Here's how the part is built. I have some questions about the finished solid (model axes, mm). A direction names the side the tool comes from. Round coordinates to 2 decimals unless told otherwise and drop trailing zeros. Write each loop counter-clockwise with the first axis right and the second up, starting at its lowest first coordinate (ties: lowest second). Pieces come first, ordered by that corner, then holes. Notation, with made-up numbers: (34, 67.5) - (63, 67.5) arc R31 cw to (63, 97.5) - close; hole circle Ø10 at (-25.75, 76.25). An arc over 180 degrees is marked (long way). One line per question, with ' | ' between items. Start each with the question number.
(1) For faces 3 (the flat face through (0, 25, 0.5)), 4 (the cylindrical face through (-2.38, 40.74, -1.27)), 5 (the flat face through (7, 35, -2.5)), 6 (the flat face through (5, -1, -2)), which set-ups out of +Z, -Z, +X, -X, +Y, -Y let a thin tool reach every point of the face, with its end or its side?
(2) Imagine slicing it at B-B (y = -26.6). Write out the boundary of the cut face in (x, z).
(3) Imagine slicing it at C-C (y = 16). Write out the boundary of the cut face in (x, z), plus the area to 3 significant figures.
(4) Imagine slicing it at D-D (x = -2). Write out the boundary of the cut face in (y, z), plus the area to 3 significant figures.
(5) Imagine slicing it at A-A (z = 4.25). Write out the boundary of the cut face in (x, y).
(6) Will these pins go through, and if not, where does the flat tip stop? pin 1 (4.5 mm diameter, centred on x = -8, y = -26.6, fed in from -Z); pin 2 (0.6 mm diameter, centred on x = 3.5, z = 0.5, fed in from +Y); pin 3 (2.5 mm diameter, centred on x = 5.66, y = 35.66, fed in from -Z); pin 4 (2.5 mm diameter, centred on x = -5.66, y = 35.66, fed in from +Z).
(7) If I drill on L1, parallel to Y at x = 0, z = 0.3; L2, parallel to Y at x = -0.75, z = -0.5; L3, parallel to Y at x = -1.5, z = 2, over which ranges is the centre line in solid material (lowest first)?
(8) Thinking about a two-plate mould opening in Y: for faces 1 (the flat face through (-0.2, -28.3, 5)), 2 (the cylindrical face through (-0.1, 18.5, -1.5)), which applies, pulls with the +Y half, pulls with the -Y half, needs draft (parallel to the pull), parting line crosses it, or undercut?
from build123d import *
from build123d.topology import SkipClean

# Parameters (mm, degrees)
BOSS_EXTRUDE1_DEPTH           = 3
BOSS_EXTRUDE2_START           = -0.5
SKETCH1_3_R                   = 11
BOSS_EXTRUDE2_DEPTH           = 0.5
SKETCH2_R                     = 4.1
SKETCH2_R_2                   = 1.1
CUT_EXTRUDE1_DEPTH            = 3.5
SKETCH2_3_R                   = 2
CUT_EXTRUDE2_DEPTH            = 0.5
CIRPATTERN2_COUNT             = 4
SKETCH1_6_W                   = 11
SKETCH1_6_H                   = 6
BOSS_EXTRUDE3_DEPTH           = 5
SKETCH4_R                     = 1.35
CUT_EXTRUDE4_DEPTH            = 8
LPATTERN2_COUNT               = 2
LPATTERN2_PITCH               = 8
LPATTERN2_COL_COUNT           = 2
LPATTERN2_COL_PITCH           = 8
BODY_MOVE_COPY1_START         = -3
BODY_MOVE_COPY1_OUTLINE_R     = 2
BODY_MOVE_COPY1_OUTLINE_R_2   = 4.1
BODY_MOVE_COPY1_DEPTH         = 3
BODY_MOVE_COPY1_START_2       = 3
BODY_MOVE_COPY1_2_OUTLINE_W   = 22
BODY_MOVE_COPY1_2_OUTLINE_H   = 6
BODY_MOVE_COPY1_2_OUTLINE_R   = 1.35
BODY_MOVE_COPY1_2_DEPTH       = 2
BODY_MOVE_COPY1_START_3       = -2.5
BODY_MOVE_COPY1_3_OUTLINE_R   = 2
BODY_MOVE_COPY1_3_OUTLINE_R_2 = 1.1
BODY_MOVE_COPY1_3_DEPTH       = 2
BODY_MOVE_COPY1_START_4       = 0.5
BODY_MOVE_COPY1_4_OUTLINE_R   = 1.1
BODY_MOVE_COPY1_4_OUTLINE_R_2 = 4.1
BODY_MOVE_COPY1_4_DEPTH       = 2.5
BODY_MOVE_COPY1_5_DEPTH       = 0.5
BODY_MOVE_COPY1_START_5       = -5
BODY_MOVE_COPY1_6_OUTLINE_W   = 22
BODY_MOVE_COPY1_6_OUTLINE_H   = 6
BODY_MOVE_COPY1_6_OUTLINE_R   = 1.35
BODY_MOVE_COPY1_6_DEPTH       = 2


# Read off the part's stored shape, not the designer's step: Body-Move/Copy1
with BuildPart() as part:
    # Sketch1 → Boss-Extrude1 (new body)
    with BuildSketch(Plane.XY):
        with BuildLine():
            Line((-11, 30), (-11, -30))
            Line((-11, -30), (11, -30))
            Line((11, -30), (11, 30))
            ThreePointArc((11, 30), (0, 41), (-11, 30))
        make_face()
        with BuildLine():
            Line((5, -23), (-5, -23))
            Line((-5, -23), (-5, 19.643842411))
            ThreePointArc((-5, 19.643842411), (0, 18.5), (5, 19.643842411))
            Line((5, 19.643842411), (5, -23))
        make_face(mode=Mode.SUBTRACT)
    extrude(amount=BOSS_EXTRUDE1_DEPTH)

    # Sketch1<3> → Boss-Extrude2 (add)
    with BuildSketch(Plane.XY.offset(BOSS_EXTRUDE2_START)):
        with Locations((0, 30)):
            Circle(SKETCH1_3_R)
    extrude(amount=BOSS_EXTRUDE2_DEPTH)

    # Sketch2 → Cut-Extrude1 (cut)
    with BuildSketch(Plane.XY.offset(3)):
        with Locations((0, 30)):
            Circle(SKETCH2_R)
        with Locations((5.656854249, 35.656854249)):
            Circle(SKETCH2_R_2)
    cut_extrude1 = extrude(amount=-CUT_EXTRUDE1_DEPTH, mode=Mode.SUBTRACT)

    # Sketch2<3> → Cut-Extrude2 (cut)
    with BuildSketch(Plane.XY.offset(3)):
        with Locations((5.656854249, 35.656854249)):
            Circle(SKETCH2_3_R)
    cut_extrude2 = extrude(amount=-CUT_EXTRUDE2_DEPTH, mode=Mode.SUBTRACT)

    # CirPattern2: Cut-Extrude1, Cut-Extrude2 ×4 about axis
    cirpattern2_axis = Axis((0, 30, 0), (0, 0, 1))
    add([cut_extrude1.rotate(cirpattern2_axis, i * 360 / CIRPATTERN2_COUNT) for i in range(1, CIRPATTERN2_COUNT)], mode=Mode.SUBTRACT)
    add([cut_extrude2.rotate(cirpattern2_axis, i * 360 / CIRPATTERN2_COUNT) for i in range(1, CIRPATTERN2_COUNT)], mode=Mode.SUBTRACT)

    # Sketch1<6> → Boss-Extrude3 (add)
    with BuildSketch(Plane.XY):
        with Locations((-5.5, -27)):
            Rectangle(SKETCH1_6_W, SKETCH1_6_H)
        with Locations((5.5, -27)):
            Rectangle(SKETCH1_6_W, SKETCH1_6_H)
    extrude(amount=-BOSS_EXTRUDE3_DEPTH)

    # Sketch4 → Cut-Extrude4 (cut)
    with BuildSketch(Plane.XY.offset(3)):
        with Locations((0, -26.6)):
            Circle(SKETCH4_R)
    cut_extrude4 = extrude(amount=-CUT_EXTRUDE4_DEPTH, mode=Mode.SUBTRACT)

    # LPattern2: Cut-Extrude4 ×2
    with Locations(*[(i * LPATTERN2_PITCH, 0, 0) for i in range(1, LPATTERN2_COUNT)]):
        add(cut_extrude4, mode=Mode.SUBTRACT)

    # LPattern2 col: Cut-Extrude4 ×2
    with Locations(*[(-i * LPATTERN2_COL_PITCH, 0, 0) for i in range(1, LPATTERN2_COL_COUNT)]):
        add(cut_extrude4, mode=Mode.SUBTRACT)

    # Body-Move/Copy1 outline → Body-Move/Copy1 (add)
    with BuildSketch(Plane.XY.offset(BODY_MOVE_COPY1_START)):
        with BuildLine():
            Line((-11, -24), (11, -24))
            Line((11, -24), (11, 30))
            ThreePointArc((11, 30), (0, 41), (-11, 30))
            Line((-11, 30), (-11, -24))
        make_face()
        with BuildLine():
            Line((5, 19.643842411), (5, -23))
            Line((5, -23), (-5, -23))
            Line((-5, -23), (-5, 19.643842411))
            ThreePointArc((-5, 19.643842411), (0, 18.5), (5, 19.643842411))
        make_face(mode=Mode.SUBTRACT)
        with Locations((5.656854249, 35.656854249)):
            Circle(BODY_MOVE_COPY1_OUTLINE_R, mode=Mode.SUBTRACT)
        with Locations((-5.656854249, 24.343145751)):
            Circle(BODY_MOVE_COPY1_OUTLINE_R, mode=Mode.SUBTRACT)
        with Locations((-5.656854249, 35.656854249)):
            Circle(BODY_MOVE_COPY1_OUTLINE_R, mode=Mode.SUBTRACT)
        with Locations((0, 30)):
            Circle(BODY_MOVE_COPY1_OUTLINE_R_2, mode=Mode.SUBTRACT)
        with Locations((5.656854249, 24.343145751)):
            Circle(BODY_MOVE_COPY1_OUTLINE_R, mode=Mode.SUBTRACT)
    extrude(amount=BODY_MOVE_COPY1_DEPTH)

    # Body-Move_Copy1 2 outline → Body-Move_Copy1 2 (add)
    with BuildSketch(Plane.XY.offset(BODY_MOVE_COPY1_START_2)):
        with Locations((0, -27)):
            Rectangle(BODY_MOVE_COPY1_2_OUTLINE_W, BODY_MOVE_COPY1_2_OUTLINE_H)
        with Locations((-8, -26.6)):
            Circle(BODY_MOVE_COPY1_2_OUTLINE_R, mode=Mode.SUBTRACT)
        with Locations((0, -26.6)):
            Circle(BODY_MOVE_COPY1_2_OUTLINE_R, mode=Mode.SUBTRACT)
        with Locations((8, -26.6)):
            Circle(BODY_MOVE_COPY1_2_OUTLINE_R, mode=Mode.SUBTRACT)
    extrude(amount=BODY_MOVE_COPY1_2_DEPTH)

    # Body-Move_Copy1 3 outline → Body-Move_Copy1 3 (add)
    # profile 1 of 4: a face of its own
    with BuildSketch(Plane.XY.offset(BODY_MOVE_COPY1_START_3)):
        with Locations((5.656854249, 35.656854249)):
            Circle(BODY_MOVE_COPY1_3_OUTLINE_R)
        with Locations((5.656854249, 35.656854249)):
            Circle(BODY_MOVE_COPY1_3_OUTLINE_R_2, mode=Mode.SUBTRACT)
    # profile 2 of 4: a face of its own
    with BuildSketch(Plane.XY.offset(BODY_MOVE_COPY1_START_3)):
        with Locations((5.656854249, 24.343145751)):
            Circle(BODY_MOVE_COPY1_3_OUTLINE_R)
        with Locations((5.656854249, 24.343145751)):
            Circle(BODY_MOVE_COPY1_3_OUTLINE_R_2, mode=Mode.SUBTRACT)
    # profile 3 of 4: a face of its own
    with BuildSketch(Plane.XY.offset(BODY_MOVE_COPY1_START_3)):
        with Locations((-5.656854249, 35.656854249)):
            Circle(BODY_MOVE_COPY1_3_OUTLINE_R)
        with Locations((-5.656854249, 35.656854249)):
            Circle(BODY_MOVE_COPY1_3_OUTLINE_R_2, mode=Mode.SUBTRACT)
    # profile 4 of 4: a face of its own
    with BuildSketch(Plane.XY.offset(BODY_MOVE_COPY1_START_3)):
        with Locations((-5.656854249, 24.343145751)):
            Circle(BODY_MOVE_COPY1_3_OUTLINE_R)
        with Locations((-5.656854249, 24.343145751)):
            Circle(BODY_MOVE_COPY1_3_OUTLINE_R_2, mode=Mode.SUBTRACT)
    extrude(amount=BODY_MOVE_COPY1_3_DEPTH)

    # Body-Move_Copy1 4 outline → Body-Move_Copy1 4 (cut)
    with BuildSketch(Plane.XY.offset(BODY_MOVE_COPY1_START_4)):
        with BuildLine():
            ThreePointArc((11, 30), (0, 41), (-11, 30))
            Line((-11, 30), (-11, -24))
            Line((-11, -24), (11, -24))
            Line((11, -24), (11, 30))
        make_face()
        with Locations((5.656854249, 35.656854249)):
            Circle(BODY_MOVE_COPY1_4_OUTLINE_R, mode=Mode.SUBTRACT)
        with Locations((0, 30)):
            Circle(BODY_MOVE_COPY1_4_OUTLINE_R_2, mode=Mode.SUBTRACT)
        with BuildLine():
            Line((5, -23), (-5, -23))
            Line((-5, -23), (-5, 19.643842411))
            ThreePointArc((-5, 19.643842411), (0, 18.5), (5, 19.643842411))
            Line((5, 19.643842411), (5, -23))
        make_face(mode=Mode.SUBTRACT)
        with Locations((-5.656854249, 24.343145751)):
            Circle(BODY_MOVE_COPY1_4_OUTLINE_R, mode=Mode.SUBTRACT)
        with Locations((-5.656854249, 35.656854249)):
            Circle(BODY_MOVE_COPY1_4_OUTLINE_R, mode=Mode.SUBTRACT)
        with Locations((5.656854249, 24.343145751)):
            Circle(BODY_MOVE_COPY1_4_OUTLINE_R, mode=Mode.SUBTRACT)
    extrude(amount=BODY_MOVE_COPY1_4_DEPTH, mode=Mode.SUBTRACT)

    # Body-Move_Copy1 5 outline → Body-Move_Copy1 5 (cut)
    with SkipClean():  # the faces are left unmerged after this step: merging them gives an invalid solid
        with BuildSketch(Plane.XY):
            with BuildLine():
                Line((-11, -24), (11, -24))
                Line((11, -24), (11, 30))
                ThreePointArc((11, 30), (0, 19), (-11, 30))
                Line((-11, 30), (-11, -24))
            make_face()
            with BuildLine():
                Line((5, 19.643842411), (5, -23))
                Line((5, -23), (-5, -23))
                Line((-5, -23), (-5, 19.643842411))
                ThreePointArc((-5, 19.643842411), (0, 18.5), (5, 19.643842411))
            make_face(mode=Mode.SUBTRACT)
        extrude(amount=BODY_MOVE_COPY1_5_DEPTH, mode=Mode.SUBTRACT)
    add(part.part.scale(1), mode=Mode.REPLACE)  # the faces are merged on a copy

    # Body-Move_Copy1 6 outline → Body-Move_Copy1 6 (cut)
    with BuildSketch(Plane.XY.offset(BODY_MOVE_COPY1_START_5)):
        with Locations((0, -27)):
            Rectangle(BODY_MOVE_COPY1_6_OUTLINE_W, BODY_MOVE_COPY1_6_OUTLINE_H)
        with Locations((-8, -26.6)):
            Circle(BODY_MOVE_COPY1_6_OUTLINE_R, mode=Mode.SUBTRACT)
        with Locations((0, -26.6)):
            Circle(BODY_MOVE_COPY1_6_OUTLINE_R, mode=Mode.SUBTRACT)
        with Locations((8, -26.6)):
            Circle(BODY_MOVE_COPY1_6_OUTLINE_R, mode=Mode.SUBTRACT)
    extrude(amount=BODY_MOVE_COPY1_6_DEPTH, mode=Mode.SUBTRACT)


solid = part.part
Check sheet entries:
1) face 3: +Z, +X, -X, +Y | face 4: +Z | face 5: -Z | face 6: +Z, -Z
2) outline: (-11, -3) - (-9.35, -3) - (-9.35, 5) - (-11, 5) - close; (-6.65, -3) - (-1.35, -3) - (-1.35, 5) - (-6.65, 5) - close; (1.35, -3) - (6.65, -3) - (6.65, 5) - (1.35, 5) - close; (9.35, -3) - (11, -3) - (11, 5) - (9.35, 5) - close
3) outline: (-11, -3) - (-5, -3) - (-5, 0) - (-11, 0) - close; (5, -3) - (11, -3) - (11, 0) - (5, 0) - close | area: 36.0 mm^2
4) outline: (-30, -3) - (-23, -3) - (-23, 0) - (-24, 0) - (-24, 5) - (-30, 5) - close; (18.68, -3) - (26.42, -3) - (26.42, 0.5) - (19.18, 0.5) - (19.18, 0) - (18.68, 0) - close; (33.58, -3) - (40.82, -3) - (40.82, 0.5) - (33.58, 0.5) - close | area: 103 mm^2
5) outline: (-11, -30) - (11, -30) - (11, -24) - (-11, -24) - close; hole circle Ø2.7 at (-8, -26.6); hole circle Ø2.7 at (0, -26.6); hole circle Ø2.7 at (8, -26.6)
6) pin 1: z = -3 | pin 2: y = 40.52 | pin 3: z = -2.5 | pin 4: z = 0.5
7) L1: -30 to -27.95, -25.25 to -24, 19 to 25.9, 34.1 to 41 | L2: -30 to -27.72, -25.48 to -23, 18.52 to 25.97, 34.03 to 40.97 | L3: -30 to -24
8) face 1: needs draft | face 2: undercut
